Can you work these out from the model? Positions are in its coordinate system, mm. Round coordinates to 2 decimals unless told otherwise and drop trailing zeros. Loops run counter-clockwise (first coordinate to the right, second up) from the corner with the lowest first, then second, coordinate; pieces in that order, holes last. Notation, with made-up numbers: M 9.5,30 L 48.5,30 A30 cw 48.5,64 Z; hole C 48,43.25 d11. An arc over 180 degrees is marked long. Use a Markdown table: item, result. Add a question column.
```python
from build123d import *

# Parameters (mm, degrees)
ESQUISSE1_W             = 30
ESQUISSE1_H             = 9
BOSS_EXTRU_1_DEPTH      = 5.5
ESQUISSE3_R             = 1
ENL_V_MAT_EXTRU_2_DEPTH = 6.5
ESQUISSE4_R             = 1.5
ENL_V_MAT_EXTRU_3_DEPTH = 10


with BuildPart() as part:
    # Esquisse1 → Boss.-Extru.1 (new body)
    with BuildSketch(Plane.XY):
        with Locations((-4.19131449, -1.696581197)):
            Rectangle(ESQUISSE1_W, ESQUISSE1_H)
    extrude(amount=BOSS_EXTRU_1_DEPTH)

    # Esquisse3 → Enlèv. mat.-Extru.2 (cut, through all)
    with BuildSketch(Plane.XY.offset(5.5)):
        with Locations((6.30868551, 0.303418803)):
            Circle(ESQUISSE3_R)
        with Locations((-1.69131449, 0.303418803)):
            Circle(ESQUISSE3_R)
        with Locations((-9.69131449, 0.303418803)):
            Circle(ESQUISSE3_R)
    extrude(amount=-ENL_V_MAT_EXTRU_2_DEPTH, mode=Mode.SUBTRACT)

    # Esquisse4 → Enlèv. mat.-Extru.3 (cut)
    with BuildSketch(Plane.XY.offset(5.5)):
        with Locations((-7.19131449, -4.196581197)):
            Circle(ESQUISSE4_R)
        with Locations((7.80868551, -4.196581197)):
            Circle(ESQUISSE4_R)
    extrude(amount=-ENL_V_MAT_EXTRU_3_DEPTH, mode=Mode.SUBTRACT)


solid = part.part
```
(1) If I drill on probe 1 along Y at (x, z) = (-9.75, 2.7); probe 2 along X at (y, z) = (-5.5, 1.55); probe 3 along X at (y, z) = (-0.25, 1.6), over which ranges is the centre line in solid material (lowest first)? Write a range as [from, to].
(2) Suppose I cut it at D-D on y = -3.5. List the corners of the cut face in (x, z) for me.
(3) Suppose I cut it at A-A on x = 5.75. List the corners of the cut face in (y, z) for me, and give its area (3 significant figures).
(4) Suppose I cut it at C-C on z = 1.35. List the corners of the cut face in (x, y) for me, and give its area (3 significant figures).
(5) Thinking about a two-plate mould opening in X: for faces 1 (the face through (-4, -2, 5.5)), 2 (the face through (-0.737, 0.604, 2.788)), 3 (the face through (-19.191, -2, 3)), which applies, released by +X, released by -X, zero draft, split by the parting line, or undercut?
(6) Suppose I cut it at B-B on y = 0.75. List the corners of the cut face in (x, z) for me.
Results below:
| question | item | result |
|---|---|---|
| 1 | probe 1 | y = [-6.2, -0.69], [1.3, 2.8] |
| 1 | probe 2 | x = [-19.19, -7.93], [-6.45, 7.07], [8.55, 10.81] |
| 1 | probe 3 | x = [-19.19, -10.52], [-8.86, -2.52], [-0.86, 5.48], [7.14, 10.81] |
| 2 | outline | M -19.19,0 L -8.52,0 L -8.52,5.5 L -19.19,5.5 Z; M -5.86,0 L 6.48,0 L 6.48,5.5 L -5.86,5.5 Z; M 9.14,0 L 10.81,0 L 10.81,5.5 L 9.14,5.5 Z |
| 3 | outline | M -6.2,0 L -0.53,0 L -0.53,5.5 L -6.2,5.5 Z; M 1.13,0 L 2.8,0 L 2.8,5.5 L 1.13,5.5 Z |
| 3 | area | 40.4 mm² |
| 4 | outline | M -19.19,-6.2 L 10.81,-6.2 L 10.81,2.8 L -19.19,2.8 Z; hole C -9.69,0.3 d2; hole C -7.19,-4.2 d3; hole C -1.69,0.3 d2; hole C 6.31,0.3 d2; hole C 7.81,-4.2 d3 |
| 4 | area | 246 mm² |
| 5 | face 1 | zero draft |
| 5 | face 2 | undercut |
| 5 | face 3 | released by -X |
| 6 | outline | M -19.19,0 L -10.59,0 L -10.59,5.5 L -19.19,5.5 Z; M -8.8,0 L -2.59,0 L -2.59,5.5 L -8.8,5.5 Z; M -0.8,0 L 5.41,0 L 5.41,5.5 L -0.8,5.5 Z; M 7.2,0 L 10.81,0 L 10.81,5.5 L 7.2,5.5 Z |
